Could you check a few things on this drawing? It's one solid part, dimensions in mm from its lowest x, y, z. Give positions to 0.01 mm unless a question says otherwise; leave off trailing zeros. Order: outer loops, then holes, each group sorted by start corner. A loop starts at its lowest first (then second) coordinate and runs counter-clockwise, first axis right, second up. Notation, with made-up numbers: (82, 8) - (116, 8) arc R12 cw to (116, 15) - close; hole circle Ø7 at (10, -8). An arc over 180 degrees is marked (long way). Answer as CSV lines item,"result".
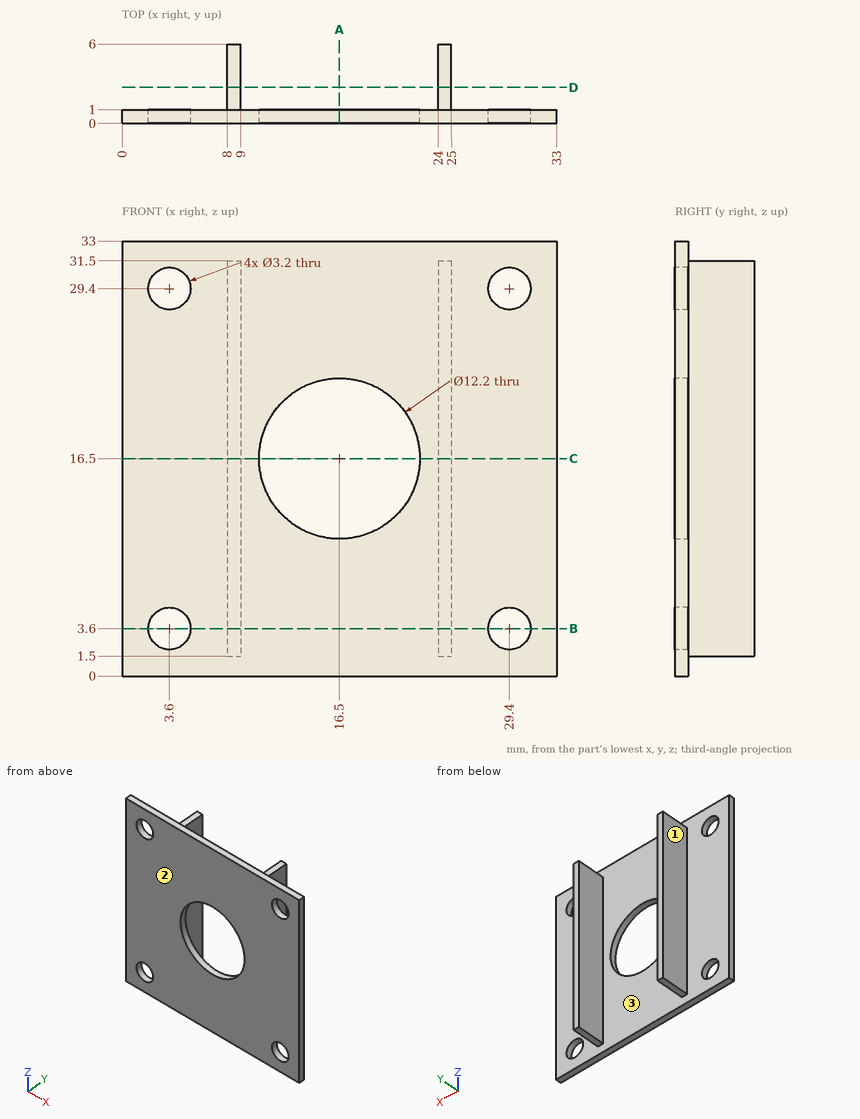
1) I need wall thicknesses on line 1 along X through (y, z) = (0.2, 29.4); line 2 along X through (y, z) = (5.35, 20); line 3 along X through (y, z) = (0.6, 16.5). Which ranges of each line are inside material? Lowest first, please. Write a range as [from, to].
Answer block:
line 1,"[0, 2], [5.2, 27.8], [31, 33]"
line 2,"[8, 9], [24, 25]"
line 3,"[0, 10.4], [22.6, 33]"
2) If we mould it in two halves opening along X, with no side actions, what happens to the marked faces 1, 2 and 3? For each: +X half, -X half, draft (parallel to the pull), parting line (faces both ways), or undercut.
Answer block:
face 1,"-X half"
face 2,"draft"
face 3,"undercut"
3) I want a section at B-B on z = 3.6. Write out the boundary of the cut face in (x, y), plus the area to 3 significant figures.
Answer block:
outline,"(0, 0) - (2, 0) - (2, 1) - (0, 1) - close; (5.2, 0) - (27.8, 0) - (27.8, 1) - (25, 1) - (25, 6) - (24, 6) - (24, 1) - (9, 1) - (9, 6) - (8, 6) - (8, 1) - (5.2, 1) - close; (31, 0) - (33, 0) - (33, 1) - (31, 1) - close"
area,"36.6 mm2"
4) I want a section at C-C on z = 16.5. Write out the boundary of the cut face in (x, y).
Answer block:
outline,"(0, 0) - (10.4, 0) - (10.4, 1) - (9, 1) - (9, 6) - (8, 6) - (8, 1) - (0, 1) - close; (22.6, 0) - (33, 0) - (33, 1) - (25, 1) - (25, 6) - (24, 6) - (24, 1) - (22.6, 1) - close"
5) I want a section at D-D on y = 2.7. Write out the boundary of the cut face in (x, z), plus the area to 3 significant figures.
Answer block:
outline,"(8, 1.5) - (9, 1.5) - (9, 31.5) - (8, 31.5) - close; (24, 1.5) - (25, 1.5) - (25, 31.5) - (24, 31.5) - close"
area,"60.0 mm2"
6) I'm going to push flat-ended pins straight in: P1, Ø3, axis at x = 18.5, y = 3.5, coming from the -Z side; P2, Ø2.5, axis at y = 4, z = 19.5, coming from the -X side; P3, Ø1.5, axis at y = 4, z = 24, coming from the +X side; P4, Ø3.5, axis at x = 29.4, z = 3.6, coming from the +Y side. Where does each tip first touch, or does it pass through?
Answer block:
P1,"through"
P2,"x = 8"
P3,"x = 25"
P4,"y = 1"
7) I want a section at A-A on x = 16.5. Write out the boundary of the cut face in (y, z), plus the area to 3 significant figures.
Answer block:
outline,"(0, 0) - (1, 0) - (1, 10.4) - (0, 10.4) - close; (0, 22.6) - (1, 22.6) - (1, 33) - (0, 33) - close"
area,"20.8 mm2"
